from build123d import *

# Parameters (mm, degrees)
F0_W      = 45
F0_H      = 10
F1_DEPTH  = 23
F2_W      = 30
F2_H      = 6.27907
F2_W_2    = 7.5
F3_DEPTH  = 12.5
F5_DEPTH  = 6.28007
F7_DEPTH  = 6.28007
F8_W      = 25
F8_H      = 23
F9_DEPTH  = 5
F11_DEPTH = 23.001
F12_R     = 6.25
F13_DEPTH = 10.001


with BuildPart() as f1:
    # F0 (on Front) → F1 (new body)
    with BuildSketch(Plane.XZ):
        with Locations((1.831396, -28.768687)):
            Rectangle(F0_W, F0_H)
    extrude(amount=F1_DEPTH)

    # F2 (on face) → F3 (join)
    with BuildSketch(Plane.XY.offset(-23.768687)):
        with Locations((1.831396, -3.139535)):
            Rectangle(F2_W, F2_H)
        with Locations((20.581396, -3.139535)):
            Rectangle(F2_W_2, F2_H)
        with Locations((-16.918604, -3.139535)):
            Rectangle(F2_W_2, F2_H)
    extrude(amount=F3_DEPTH)

    # F4 (on face) → F5 (cut, through all)
    with BuildSketch(Plane.XZ.offset(6.27907)):
        Polygon((16.831396, -11.268687), (24.331396, -18.768687), (24.331396, -11.268687), align=None)
    extrude(amount=-F5_DEPTH, mode=Mode.SUBTRACT)

    # F6 (on face) → F7 (cut, through all)
    with BuildSketch(Plane.XZ.offset(6.27907)):
        Polygon((-20.668604, -11.268687), (-20.668604, -18.768687), (-13.168604, -11.268687), align=None)
    extrude(amount=-F7_DEPTH, mode=Mode.SUBTRACT)

    # F8 (on face) → F9 (cut)
    with BuildSketch(Plane(origin=(0, 0, -33.768687), x_dir=(1, 0, 0), z_dir=(0, 0, -1))):
        with Locations((1.831396, 11.5)):
            Rectangle(F8_W, F8_H)
    extrude(amount=-F9_DEPTH, mode=Mode.SUBTRACT)

    # F10 (on face) → F11 (cut, through all)
    with BuildSketch(Plane.XZ.offset(23)):
        Polygon((-10.668604, -33.768687), (-10.668604, -28.768687), (-15.668604, -28.768687), align=None)
        Polygon((19.331396, -28.768687), (14.331396, -28.768687), (14.331396, -33.768687), align=None)
    extrude(amount=-F11_DEPTH, mode=Mode.SUBTRACT)

    # F12 (on face) → F13 (cut, through all)
    with BuildSketch(Plane.XY.offset(-23.768687)):
        with Locations((1.831396, -14.639535)):
            Circle(F12_R)
    extrude(amount=-F13_DEPTH, mode=Mode.SUBTRACT)


solid = f1.part
Source: CAD feature listing. Evaluate the final solid. Frame: model axes, mm. A direction names the side the tool comes from. Coordinates: 2 decimals unless noted, no trailing zeros. Loops run counter-clockwise (first coordinate to the right, second up) from the corner with the lowest first, then second, coordinate; pieces in that order, holes last. Notation, with made-up numbers: M 65,-17.75 L 73,-17.75 A22 cw 73,7.25 Z; hole C -5.75,-10.5 d3. An arc over 180 degrees is marked long. Answer in a Markdown table with one row per item.
Q1. Section C-C on y = -18. Return the cut outline in (x, z), plus the area to 3 significant figures.
Answers below:
| item | result |
|---|---|
| outline | M -20.67,-33.77 L -10.67,-33.77 L -15.67,-28.77 L -3.44,-28.77 L -3.44,-23.77 L -20.67,-23.77 Z; M 7.1,-28.77 L 19.33,-28.77 L 14.33,-33.77 L 24.33,-33.77 L 24.33,-23.77 L 7.1,-23.77 Z |
| area | 247 mm^2 |
Q2. Section A-A on y = -3.5. Return the cut outline in (x, z), plus the area to 3 significant figures.
Answers below:
| item | result |
|---|---|
| outline | M -20.67,-33.77 L -10.67,-33.77 L -15.67,-28.77 L 19.33,-28.77 L 14.33,-33.77 L 24.33,-33.77 L 24.33,-18.77 L 16.83,-11.27 L -13.17,-11.27 L -20.67,-18.77 Z |
| area | 806 mm^2 |
Q3. Set-up query: faces 1 (the flat face through (-13.204, -11.661, -31.234)), 2 (the flat face through (2, -3, -11.269)), 3 (the flat face through (-3.5, -18.2, -23.769)). Return all of +Z, -Z, +X, -X, +Y, -Y with unobstructed straight access to the full face (end or side cutting, diameter ignored); none if empty.
Answers below:
| item | result |
|---|---|
| face 1 | +Y, -Y |
| face 2 | +Z, +X, -X, +Y, -Y |
| face 3 | +Z, +X, -X, -Y |
Q4. Section B-B on x = 0.5. Return the cut outline in (y, z), plus the area to 3 significant figures.
Answers below:
| item | result |
|---|---|
| outline | M -23,-28.77 L -20.75,-28.77 L -20.75,-23.77 L -23,-23.77 Z; M -8.53,-28.77 L 0,-28.77 L 0,-11.27 L -6.28,-11.27 L -6.28,-23.77 L -8.53,-23.77 Z |
| area | 132 mm^2 |
Q5. Section D-D on z = -29.75. Return the cut outline in (x, y).
Answers below:
| item | result |
|---|---|
| outline | M -20.67,-23 L -14.69,-23 L -14.69,0 L -20.67,0 Z; M 18.35,-23 L 24.33,-23 L 24.33,0 L 18.35,0 Z |
Q6. Ray query, probe 1 along X at (y, z) = (-14.5, -28.5); probe 2 along Y at (x, z) = (17.5, -23.5); probe 3 along Z at (x, y) = (13.5, -10.5). Return the intervals inside material, ascending. Write a range as from..to.
Answers below:
| item | result |
|---|---|
| probe 1 | x = -20.67..-4.42, 8.08..24.33 |
| probe 2 | y = -6.28..0 |
| probe 3 | z = -28.77..-23.77 |
Q7. Draft query along X for faces 4 (the flat face through (20.53, -3.18, -14.97)), 5 (the flat face through (2, -23, -28)), 6 (the flat face through (6, -9, -28.769)), 7 (the flat face through (-20.669, -12, -28)). Return one class per face: pulls with the +X half, pulls with the -X half, needs draft (parallel to the pull), parting line crosses it, or undercut.
Answers below:
| item | result |
|---|---|
| face 4 | pulls with the +X half |
| face 5 | needs draft |
| face 6 | undercut |
| face 7 | pulls with the -X half |
Q8. First-contact query: pin 1 (7.5 mm diameter, centred on x = 1.83, y = -14.64, fed in from +Z); pin 2 (1 mm diameter, centred on x = 19.5, y = -18.5, fed in from +Z); pin 3 (11.5 mm diameter, centred on x = 1.5, y = -6.5, fed in from -Z); pin 4 (6 mm diameter, centred on x = 11.5, z = -19, fed in from -Y). Flat tips, straight axial feed; report the tip coordinate or a pass-through.
Answers below:
| item | result |
|---|---|
| pin 1 | passes through |
| pin 2 | stops at z = -23.77 |
| pin 3 | stops at z = -28.77 |
| pin 4 | stops at y = -6.28 |
